Verification items for the finished model (mm, model axes). Face numbers are marked on the shaded views. A direction names the side the tool comes from. Give positions to 0.01 mm unless a question says otherwise; leave off trailing zeros. Write each loop counter-clockwise with the first axis right and the second up, starting at its lowest first coordinate (ties: lowest second). Pieces come first, ordered by that corner, then holes.
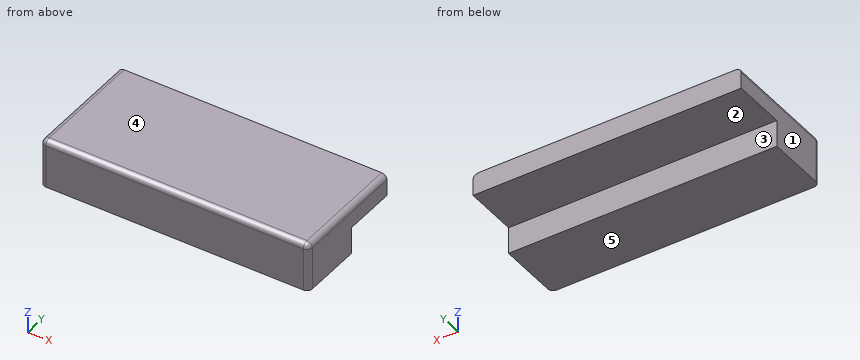
from build123d import *

# Parameters (mm, degrees)
F0_W     = 25
F0_H     = 6
F1_DEPTH = 4.5
F3_DEPTH = 5
F4_R     = 0.5
F5_R     = 0.5


with BuildPart() as f1:
    # F0 (on Top) → F1 (new body)
    with BuildSketch(Plane.XY):
        Rectangle(F0_W, F0_H)
    extrude(amount=F1_DEPTH)

    # F2 (on face) → F3 (join)
    with BuildSketch(Plane(origin=(0, 3, 0), x_dir=(-1, 0, 0), z_dir=(0, 1, 0))):
        Polygon((-12.5, 4.5), (-12.5, 2.5), (10.169396, 2.5), (12.5, 2.5), (12.5, 4.5), align=None)
    extrude(amount=F3_DEPTH)

    # F4
    f4_edges = [f1.edges().sort_by_distance(p)[0] for p in [
        (0, -3, 4.5),
    ]]
    fillet(f4_edges, radius=F4_R)

    # F5
    f5_edges = [f1.edges().sort_by_distance(p)[0] for p in [
        (12.5, 2.75, 4.5),
        (-12.5, 2.75, 4.5),
    ]]
    fillet(f5_edges, radius=F5_R)


solid = f1.part
Item 1: Sectioned sample at C-C on z = 0.55. Record the cut outline in (x, y).
Answer key:
outline: (-12.5, -2.5) arc R0.5 ccw to (-12, -3) - (12, -3) arc R0.5 ccw to (12.5, -2.5) - (12.5, 3) - (-12.5, 3) - close
Item 2: Depth check by flat-ended pin: pin 1 (1 mm diameter, centred on x = -6.5, y = 0, fed in from -Z); pin 2 (4 mm diameter, centred on x = 0, y = 6, fed in from -Z). Enter the tip coordinate at first touch or a pass-through.
Answer key:
pin 1: stops at z = 0
pin 2: stops at z = 2.5
Item 3: Sectioned sample at B-B on y = 6.25. Record the cut outline in (x, z), then the cut area to 3 significant figures.
Answer key:
outline: (-12.5, 2.5) - (12.5, 2.5) - (12.5, 4) arc R0.5 ccw to (12, 4.5) - (-12, 4.5) arc R0.5 ccw to (-12.5, 4) - close
area: 49.9 mm2
Item 4: Set-up check for the marked faces 1 and 2: record each of +Z, -Z, +X, -X, +Y, -Y from which the full face is reachable in a straight line by a thin tool's end or side.
Answer key:
face 1: +Z, -Z, -X, +Y, -Y
face 2: -Z, +X, -X, +Y
Item 5: Release check for a two-part mould opening along Z. For the marked faces 3, 4 and 5 record: released by +Z, released by -Z, zero draft, split by the parting line, or undercut.
Answer key:
face 3: zero draft
face 4: released by +Z
face 5: released by -Z
Item 6: Scan lines: line 1 along Z through (x, y) = (0.25, 6.25); line 2 along Y through (x, z) = (0.75, 2.35); line 3 along Y through (x, z) = (1, 4.2). Record each from-to range of solid material in increasing order.
Answer key:
line 1: z = 2.5 to 4.5
line 2: y = -3 to 3
line 3: y = -2.96 to 8
Item 7: Sectioned sample at A-A on x = 6.75. Record the cut outline in (y, z).
Answer key:
outline: (-3, 0) - (3, 0) - (3, 2.5) - (8, 2.5) - (8, 4.5) - (-2.5, 4.5) arc R0.5 ccw to (-3, 4) - close
